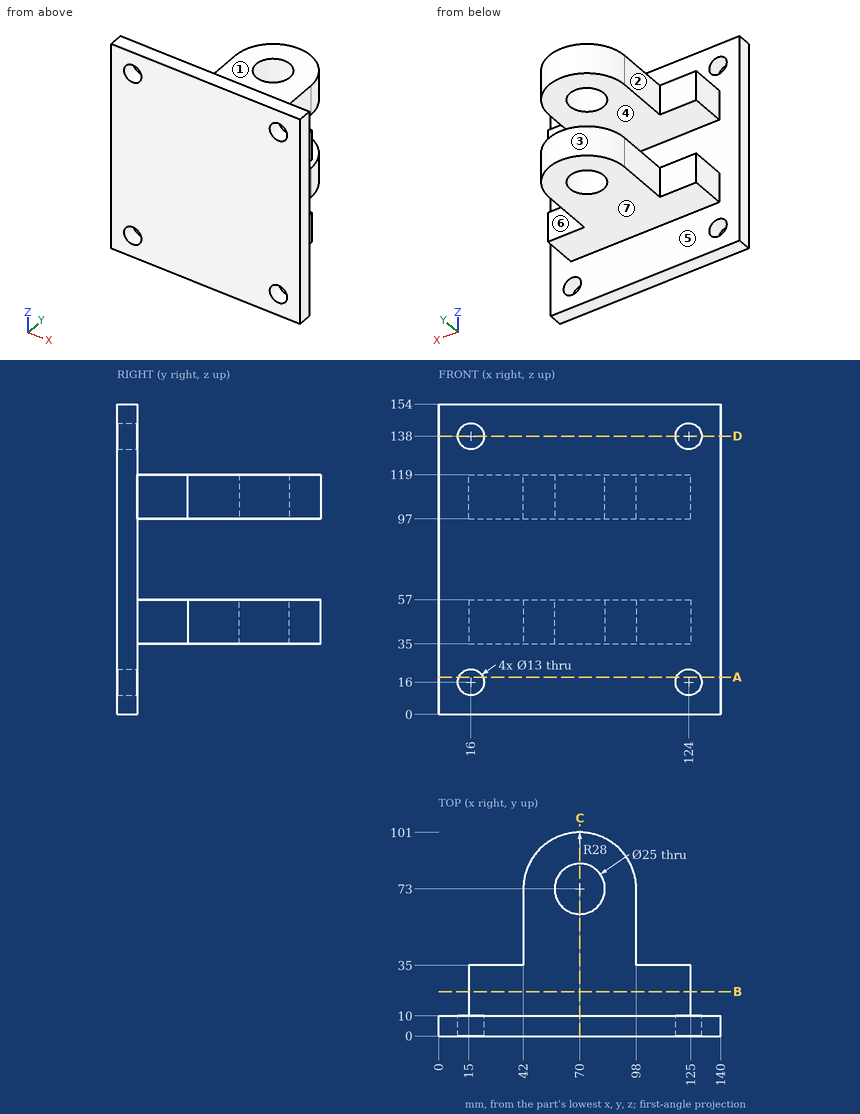
Print and shaded views of the part. All mm, measured from the part's lowest x, y and z. A direction names the side the tool comes from. Round coordinates to 2 decimals unless told otherwise and drop trailing zeros. Write each loop counter-clockwise with the first axis right and the second up, starting at its lowest first coordinate (ties: lowest second). Pieces come first, ordered by that corner, then holes. Notation, with made-up numbers: (75.25, 19) -> (106.25, 19) arc R30 cw to (106.25, 44) -> close; hole circle Ø7 at (88.5, -24). An arc over 180 degrees is marked (long way). Answer in a Markdown table with one row per item. Add a question column.
Item 1: Saw through at A-A, the plane z = 18.5. Write the cut outline in (x, y), then the cut area to 3 significant figures.
Item 2: Drill centre lines: line 1 (Z direction, x = 124, y = 7); line 2 (X direction, y = 7, z = 138); line 3 (Z direction, x = 96.5, y = 33). Where is each one in solid material? Low to high. Write a range as from..to.
Item 3: Mould opens along Z. For the marked faces 4, 5, 6 and 7 say: pulls with the +Z half, pulls with the -Z half, needs draft (parallel to the pull), parting line crosses it, or undercut.
Item 4: Saw through at C-C, the plane x = 70. Write the cut outline in (y, z).
Item 5: Which spindle directions (+Z, -Z, +X, -X, +Y, -Y) get a long thin tool onto all of the face, cutting with end or side? Do the marked faces 1, 2 and 3. Say none if no direction does.
Item 6: Saw through at D-D, the plane z = 138. Write the cut outline in (x, y), then the cut area to 3 significant figures.
Item 7: Drop flat-ended pins along their axis: pin 1 Ø12 at (x, z) = (104.5, 101) entering from +Y; pin 2 Ø15 at (x, y) = (70, 73) entering from +Z; pin 3 Ø5 at (x, z) = (38, 131) entering from +Y; pin 4 Ø10 at (y, z) = (31, 116.5) entering from +X. Give the stop position or say it passes through.
Item 8: Saw through at B-B, the plane y = 22. Write the cut outline in (x, z), then the cut area to 3 significant figures.
Findings below:
| question | item | result |
|---|---|---|
| 1 | outline | (0, 0) -> (10, 0) -> (10, 10) -> (0, 10) -> close; (22, 0) -> (118, 0) -> (118, 10) -> (22, 10) -> close; (130, 0) -> (140, 0) -> (140, 10) -> (130, 10) -> close |
| 1 | area | 1,160 mm^2 |
| 2 | line 1 | z = 0..9.5, 22.5..131.5, 144.5..154 |
| 2 | line 2 | x = 0..9.5, 22.5..117.5, 130.5..140 |
| 2 | line 3 | z = 35..57, 97..119 |
| 3 | face 4 | undercut |
| 3 | face 5 | undercut |
| 3 | face 6 | needs draft |
| 3 | face 7 | pulls with the -Z half |
| 4 | outline | (0, 0) -> (10, 0) -> (10, 35) -> (60.5, 35) -> (60.5, 57) -> (10, 57) -> (10, 97) -> (60.5, 97) -> (60.5, 119) -> (10, 119) -> (10, 154) -> (0, 154) -> close; (85.5, 35) -> (101, 35) -> (101, 57) -> (85.5, 57) -> close; (85.5, 97) -> (101, 97) -> (101, 119) -> (85.5, 119) -> close |
| 5 | face 1 | +Z, +X, -X, +Y |
| 5 | face 2 | +Z, -Z, -X, +Y |
| 5 | face 3 | +Z, -Z, +Y |
| 6 | outline | (0, 0) -> (9.5, 0) -> (9.5, 10) -> (0, 10) -> close; (22.5, 0) -> (117.5, 0) -> (117.5, 10) -> (22.5, 10) -> close; (130.5, 0) -> (140, 0) -> (140, 10) -> (130.5, 10) -> close |
| 6 | area | 1,140 mm^2 |
| 7 | pin 1 | stops at y = 35 |
| 7 | pin 2 | passes through |
| 7 | pin 3 | stops at y = 10 |
| 7 | pin 4 | stops at x = 125 |
| 8 | outline | (15, 35) -> (125, 35) -> (125, 57) -> (15, 57) -> close; (15, 97) -> (125, 97) -> (125, 119) -> (15, 119) -> close |
| 8 | area | 4,840 mm^2 |
